Input: part model. Units: mm. Frame: model coordinates. A direction names the side the tool comes from. Round coordinates to 2 decimals unless told otherwise and drop trailing zeros. Order: outer loops, then holes, each group sorted by start corner. A loop starts at its lowest first (then second) coordinate and runs counter-clockwise, first axis right, second up.
Item 1: Line query: L1, parallel to Z at x = 8, y = 14; L2, parallel to Z at x = -3, y = 11; L3, parallel to X at y = 30, z = -106. Output: solid intervals per line, ascending.
Item 2: Reachability of faces 1 (the flat face through (21, 28, -32)), 2 (the cylindrical face through (2.17, 22.24, -127.36)) from +Z, -Z, +X, -X, +Y, -Y: full face, straight path, thin tool, end or side. Return the list, or none.
Item 3: Cut plane D-D on z = -117. Output: boundary loops of the cut face in (x, y), then the cut area to 3 significant figures.
Item 4: Cut plane A-A on x = 0. Output: boundary loops of the cut face in (y, z), then the cut area to 3 significant figures.
Item 5: Mould query, pull axis X, two halves, no side actions, for faces 3 (the flat face through (0, 32, -101.5)), 4 (the flat face through (0, 0, 2)), 5 (the flat face through (-21, 28, -32)). Classes: released by +X, released by -X, zero draft, split by the parting line, or undercut.
Item 6: First-contact query: pin 1 (8 mm diameter, centred on x = 6, z = -44, fed in from +Y); pin 2 (2 mm diameter, centred on x = -15, z = -7.5, fed in from +Y); pin 3 (8 mm diameter, centred on x = -2.5, z = 11, fed in from +Y). Flat tips, straight axial feed; report the tip coordinate or a pass-through.
Item 7: Cut plane B-B on z = 30.5. Output: boundary loops of the cut face in (x, y).
Item 8: Cut plane C-C on x = -13. Output: boundary loops of the cut face in (y, z).
```python
from build123d import *

# Parameters (mm, degrees)
STOCK_MATERIAL_DEPTH      = 21
SKETCH2_R                 = 10
POWER_PLANT_CHAMBER_DEPTH = 51
AXLE_CUTOUTS_DEPTH        = 170.107214512
AXLE_CUTOUTS_DEPTH_BACK   = 170.107214512
AXLE_LAYOUT_SKETCH_R      = 1.75


with BuildPart() as part:
    # Sketch1 → Stock Material (new, symmetric)
    with BuildSketch(Plane(origin=(0, 0, 0), x_dir=(0, 0, -1), z_dir=(1, 0, 0))):
        Polygon((-152.5, 0), (152.5, 0), (152.5, 70), (-152.5, 20), align=None)
    extrude(amount=STOCK_MATERIAL_DEPTH, both=True)

    # Sketch2 → Power Plant Chamber (cut)
    with BuildSketch(Plane(origin=(0, 0, -152.5), x_dir=(-1, 0, 0), z_dir=(0, 0, -1))):
        with Locations((0, 32)):
            Circle(SKETCH2_R)
    extrude(amount=-POWER_PLANT_CHAMBER_DEPTH, mode=Mode.SUBTRACT)

    # Axle Layout Sketch → Axle Cutouts (cut, two sides: drawn at the far end of the back side and taken through both)
    with BuildSketch(Plane(origin=(0, 0, 0), x_dir=(0, 0, -1), z_dir=(1, 0, 0)).offset(-AXLE_CUTOUTS_DEPTH_BACK)):
        with Locations((-92.5, 11)):
            Circle(AXLE_LAYOUT_SKETCH_R)
        with Locations((82.5, 14)):
            Circle(AXLE_LAYOUT_SKETCH_R)
    extrude(amount=AXLE_CUTOUTS_DEPTH + AXLE_CUTOUTS_DEPTH_BACK, mode=Mode.SUBTRACT)


solid = part.part
```
From the geometry:
1. L1: z = -152.5 to -84.25, -80.75 to 152.5
1. L2: z = -152.5 to 90.75, 94.25 to 152.5
1. L3: x = -21 to -9.8, 9.8 to 21
2. face 1: +Z, -Z, +X, +Y, -Y
2. face 2: -Z
3. outline: (-21, 0) - (21, 0) - (21, 64.18) - (-21, 64.18) - close; hole circle Ø20 at (0, 32)
3. area: 2,380 mm2
4. outline: (0, -152.5) - (22, -152.5) - (22, -101.5) - (42, -101.5) - (42, -152.5) - (70, -152.5) - (20, 152.5) - (0, 152.5) - close; hole circle Ø3.5 at (11, 92.5); hole circle Ø3.5 at (14, -82.5)
4. area: 12,700 mm2
5. face 3: undercut
5. face 4: zero draft
5. face 5: released by -X
6. pin 1: stops at y = 52.87
6. pin 2: stops at y = 46.39
6. pin 3: stops at y = 43.85
7. outline: (-21, 0) - (21, 0) - (21, 40) - (-21, 40) - close
8. outline: (0, -152.5) - (70, -152.5) - (20, 152.5) - (0, 152.5) - close; hole circle Ø3.5 at (11, 92.5); hole circle Ø3.5 at (14, -82.5)
